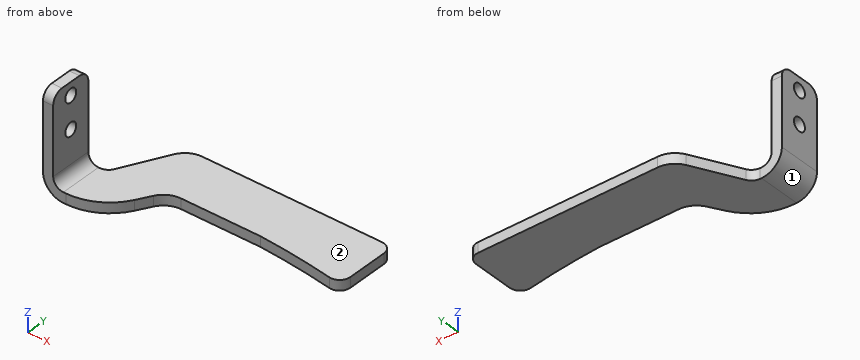
```python
from build123d import *

# Parameters (mm, degrees)
SALIENTE_EXTRUIR1_DEPTH = 6.35
CONVERTIR_S_LIDO1_DEPTH = 1.59
BRIDA_DE_ARISTA1_DEPTH  = 20
REDONDEO1_R             = 5
CORTAR_EXTRUIR1_REACH   = 138.693
CROQUIS11_R             = 3.125


# Read off the part's stored shape, not the designer's step: Convertir-Sólido1
# Sheet-metal steps are written as plain solids
with BuildPart() as part:
    # Croquis1 → Saliente-Extruir1 (new body)
    with BuildSketch(Plane.XY):
        with BuildLine():
            Line((0, 0), (1.21624327, 0))
            ThreePointArc((1.21624327, 0), (13.71624327, 3.349364905), (22.866878365, 12.5))
            Line((22.866878365, 12.5), (26.608548116, 18.980762114))
            ThreePointArc((26.608548116, 18.980762114), (30.268802154, 22.641016151), (35.268802154, 23.980762114))
            Line((35.268802154, 23.980762114), (72.43532503, 23.980762114))
            ThreePointArc((72.43532503, 23.980762114), (90.187263937, 22.435296605), (107.837539609, 19.988345998))
            ThreePointArc((107.837539609, 19.988345998), (111.885560079, 21.109920556), (113.65, 24.921895239))
            Line((113.65, 24.921895239), (113.65, 43.980762114))
            ThreePointArc((113.65, 43.980762114), (112.185533906, 47.516296019), (108.65, 48.980762114))
            Line((108.65, 48.980762114), (24.734232406, 48.980762114))
            ThreePointArc((24.734232406, 48.980762114), (19.536461106, 47.523781106), (15.853300619, 43.577396815))
            Line((15.853300619, 43.577396815), (5.048349691, 22.701682649))
            ThreePointArc((5.048349691, 22.701682649), (3.206769447, 20.728490504), (0.607883797, 20))
            Line((0.607883797, 20), (0, 20))
            Line((0, 20), (0, 0))
        make_face()
    extrude(amount=SALIENTE_EXTRUIR1_DEPTH)

    # Convertir-Sólido1 outline → Convertir-Sólido1 (cut)
    with BuildSketch(Plane.XY):
        with BuildLine():
            Line((0, 20), (0, 0))
            Line((0, 0), (1.21624327, 0))
            ThreePointArc((1.21624327, 0), (13.71624327, 3.349364905), (22.866878365, 12.5))
            Line((22.866878365, 12.5), (26.608548116, 18.980762114))
            ThreePointArc((26.608548116, 18.980762114), (30.268802154, 22.641016151), (35.268802154, 23.980762114))
            Line((35.268802154, 23.980762114), (72.43532503, 23.980762114))
            ThreePointArc((72.43532503, 23.980762114), (90.187263937, 22.435296605), (107.837539609, 19.988345998))
            ThreePointArc((107.837539609, 19.988345998), (111.885560079, 21.109920556), (113.65, 24.921895239))
            Line((113.65, 24.921895239), (113.65, 43.980762114))
            ThreePointArc((113.65, 43.980762114), (112.185533906, 47.516296019), (108.65, 48.980762114))
            Line((108.65, 48.980762114), (24.734232406, 48.980762114))
            ThreePointArc((24.734232406, 48.980762114), (19.536461106, 47.523781106), (15.853300619, 43.577396815))
            Line((15.853300619, 43.577396815), (5.048349691, 22.701682649))
            ThreePointArc((5.048349691, 22.701682649), (3.206769447, 20.728490504), (0.607883797, 20))
            Line((0.607883797, 20), (0, 20))
        make_face()
    extrude(amount=CONVERTIR_S_LIDO1_DEPTH, mode=Mode.SUBTRACT)

    # Brida de arista1 section (across the edge) → Brida de arista1 (add)
    with BuildSketch(Plane(origin=(-4.76, 20, 6.35), x_dir=(1, 0, 0), z_dir=(0, -1, 0))):
        with BuildLine():
            Line((-4.76, 4.76), (-4.76, 41.24))
            Line((-4.76, 41.24), (0, 41.24))
            Line((0, 41.24), (0, 4.76))
            ThreePointArc((0, 4.76), (1.394171722, 1.394171722), (4.76, 0))
            Line((4.76, 0), (4.76, -4.76))
            ThreePointArc((4.76, -4.76), (-1.971656557, -1.971656557), (-4.76, 4.76))
        make_face()
    extrude(amount=BRIDA_DE_ARISTA1_DEPTH)

    # Redondeo1
    redondeo1_edges = [part.edges().sort_by_distance(p)[0] for p in [
        (-7.14, 20, 47.59),
        (-7.14, 0, 47.59),
    ]]
    fillet(redondeo1_edges, radius=REDONDEO1_R)

    # Croquis11 → Cortar-Extruir1 (cut, up to next)
    with BuildSketch(Plane(origin=(-4.76, 0, 0), x_dir=(0, 0, -1), z_dir=(1, 0, 0)), mode=Mode.PRIVATE) as cortar_extruir1_sk1:
        with Locations((-41.59, 10)):
            Circle(CROQUIS11_R)
    cortar_extruir1_tool1 = extrude(cortar_extruir1_sk1.sketch, amount=-CORTAR_EXTRUIR1_REACH, mode=Mode.PRIVATE) & part.part
    # Croquis11 → Cortar-Extruir1 (cut, up to next)
    with BuildSketch(Plane(origin=(-4.76, 0, 0), x_dir=(0, 0, -1), z_dir=(1, 0, 0)), mode=Mode.PRIVATE) as cortar_extruir1_sk2:
        with Locations((-26.59, 10)):
            Circle(CROQUIS11_R)
    cortar_extruir1_tool2 = extrude(cortar_extruir1_sk2.sketch, amount=-CORTAR_EXTRUIR1_REACH, mode=Mode.PRIVATE) & part.part
    add(cortar_extruir1_tool1.solids().sort_by_distance((-4.76, 10, 41.59))[0], mode=Mode.SUBTRACT)
    add(cortar_extruir1_tool2.solids().sort_by_distance((-4.76, 10, 26.59))[0], mode=Mode.SUBTRACT)


solid = part.part
```
The model under review builds one solid part; all positions refer to its coordinate system, in mm. Face numbers are marked on the shaded views. A direction names the side the tool comes from. Round coordinates to 2 decimals unless told otherwise and drop trailing zeros. Loops run counter-clockwise (first coordinate to the right, second up) from the corner with the lowest first, then second, coordinate; pieces in that order, holes last. Notation, with made-up numbers: (-26.5, 44) -> (20.5, 44) arc R28 cw to (20.5, 81) -> close; hole circle Ø9 at (-21, 31.25). An arc over 180 degrees is marked (long way). Answer as a JSON object with one key per item and string values. Group by question number.
1) For line 1 (Y direction, x = -8, z = 41.59) (3 decimals); line 2 (X direction, y = 14.5, z = 30); line 3 (Z direction, x = 108, y = 20), list the stretches that pass through material, from the lowest coordinate up. Write a range as [from, to].
2) For pin 1 Ø2 at (y, z) = (15.5, 39) entering from +X; pin 2 Ø1.4 at (x, z) = (60.5, 5) entering from -Y; pin 3 Ø2 at (x, y) = (8, 22.5) entering from +Z; pin 4 Ø5.5 at (y, z) = (10, 26.59) entering from -X, all flat-tipped, find the tip position at first contact; note any pin that passes through.
3) We need section D-D on x = 51. Write out the cut boundary in (y, z).
4) For the marked faces 1 and 2, list the 3-axis set-ups (+Z, -Z, +X, -X, +Y, -Y) from which the entire face can be reached by the end or side of a thin tool; tool diameter is ignored.
5) We need section C-C on y = 21.5. Write out the cut boundary in (x, z).
6) We need section A-A on z = 26.59. Write out the cut boundary in (x, y) (3 decimals).
7) We need section B-B on y = 10. Write out the cut boundary in (x, z) (3 decimals).
Result set:
{
 "1": {"line 1": "[0, 6.875], [13.125, 20]", "line 2": "[-9.52, -4.76]", "line 3": "[1.59, 6.35]"},
 "2": {"pin 1": "x = -4.76", "pin 2": "y = 23.98", "pin 3": "z = 6.35", "pin 4": "through"},
 "3": {"outline": "(23.98, 1.59) -> (48.98, 1.59) -> (48.98, 6.35) -> (23.98, 6.35) -> close"},
 "4": {"face 1": "-Z, -X, +Y, -Y", "face 2": "+Z, +X, +Y, -Y"},
 "5": {"outline": "(4.18, 1.59) -> (28.68, 1.59) -> (28.68, 6.35) -> (4.18, 6.35) -> close; (97.74, 1.59) -> (112.3, 1.59) -> (112.3, 6.35) -> (97.74, 6.35) -> close"},
 "6": {"outline": "(-9.52, 0) -> (-4.76, 0) -> (-4.76, 6.875) -> (-9.52, 6.875) -> close; (-9.52, 13.125) -> (-4.76, 13.125) -> (-4.76, 20) -> (-9.52, 20) -> close"},
 "7": {"outline": "(-9.52, 11.11) arc R9.52 ccw to (0, 1.59) -> (21.216, 1.59) -> (21.216, 6.35) -> (0, 6.35) arc R4.76 cw to (-4.76, 11.11) -> (-4.76, 23.465) -> (-9.52, 23.465) -> close; (-9.52, 29.715) -> (-4.76, 29.715) -> (-4.76, 38.465) -> (-9.52, 38.465) -> close; (-9.52, 44.715) -> (-4.76, 44.715) -> (-4.76, 47.59) -> (-9.52, 47.59) -> close"}
}
